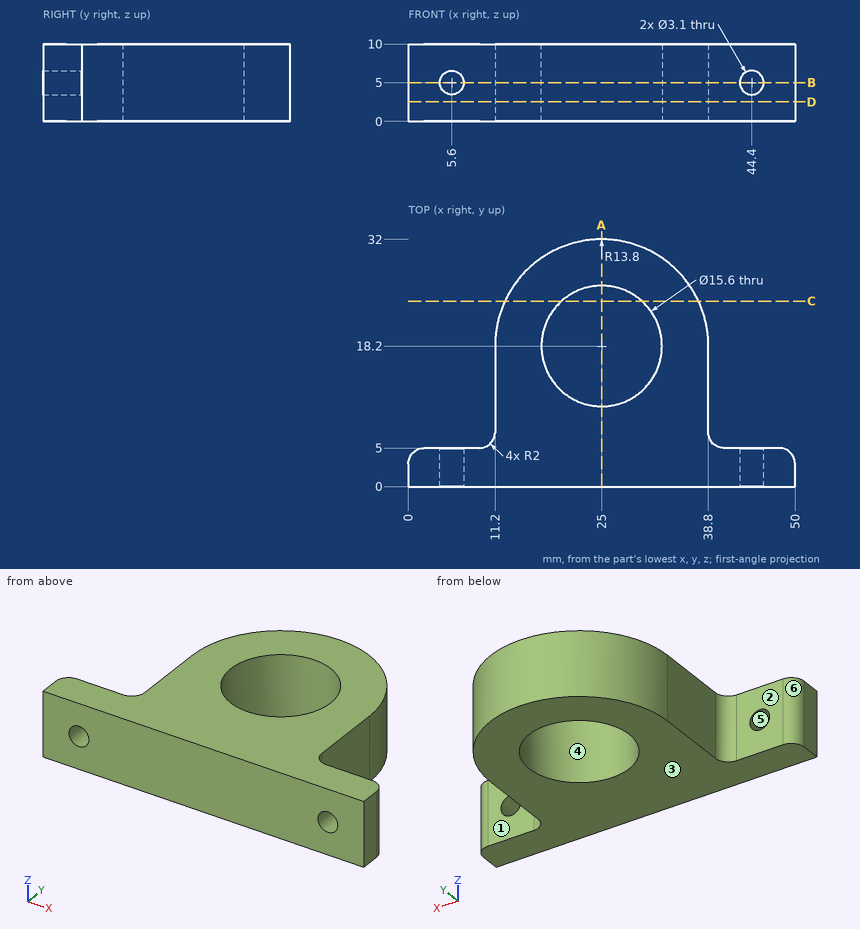
Here's the drawing with two shaded views (mm, measured from the low corner). I have some questions. A direction names the side the tool comes from. Give positions to 0.01 mm unless a question says otherwise; leave off trailing zeros. Order: outer loops, then holes, each group sorted by start corner. A loop starts at its lowest first (then second) coordinate and runs counter-clockwise, first axis right, second up. Notation, with made-up numbers: (50, 58) -> (71, 58) arc R32 ccw to (71, 95) -> close; hole circle Ø7 at (73.5, -30.75). An arc over 180 degrees is marked (long way). One line per item, written item: value. Start each with the question number.
1. Imagine slicing it at A-A, the plane x = 25. List the corners of the cut face in (y, z) for me.
2. Will these pins go through, and if not, where does the flat tip stop? pin 1 Ø1 at (y, z) = (5, 6.5) entering from -X; pin 2 Ø5 at (y, z) = (28, 6) entering from +X; pin 3 Ø3 at (y, z) = (13, 5.5) entering from -X.
3. I need wall thicknesses on probe 1 along X at (y, z) = (1.95, 5); probe 2 along Y at (x, z) = (25, 6.75); probe 3 along X at (y, z) = (18.5, 2.25). Which ranges of each line are inside material? Lowest first, please. Write a range as from..to.
4. For the marked faces 1, 2 and 3, which set-ups out of +Z, -Z, +X, -X, +Y, -Y let a thin tool reach every point of the face, with its end or its side?
5. Imagine slicing it at B-B, the plane z = 5. List the corners of the cut face in (x, y) for me, plus the area to 3 significant figures.
6. Imagine slicing it at D-D, the plane z = 2.5. List the corners of the cut face in (x, y) for me.
7. We'd pull the mould along Y, two halves only. Please class the marked faces 4, 5 and 6: released by +Y, released by -Y, zero draft, split by the parting line, or undercut.
8. Imagine slicing it at C-C, the plane y = 24. List the corners of the cut face in (x, z) for me.
Values follow:
1. outline: (0, 0) -> (10.4, 0) -> (10.4, 10) -> (0, 10) -> close; (26, 0) -> (32, 0) -> (32, 10) -> (26, 10) -> close
2. pin 1: stops at x = 0.68
2. pin 2: stops at x = 36.71
2. pin 3: stops at x = 11.2
3. probe 1: x = 0..4.05, 7.15..42.85, 45.95..50
3. probe 2: y = 0..10.4, 26..32
3. probe 3: x = 11.2..17.21, 32.79..38.8
4. face 1: +Z, -Z, +X, +Y
4. face 2: +Z, -Z, -X, +Y
4. face 3: -Z, +X, -X, +Y, -Y
5. outline: (0, 0) -> (4.05, 0) -> (4.05, 5) -> (2, 5) arc R2 ccw to (0, 3) -> close; (7.15, 0) -> (42.85, 0) -> (42.85, 5) -> (40.8, 5) arc R2 cw to (38.8, 7) -> (38.8, 18.2) arc R13.8 ccw to (11.2, 18.2) -> (11.2, 7) arc R2 cw to (9.2, 5) -> (7.15, 5) -> close; (45.95, 0) -> (50, 0) -> (50, 3) arc R2 ccw to (48, 5) -> (45.95, 5) -> close; hole circle Ø15.6 at (25, 18.2)
5. area: 691 mm2
6. outline: (0, 0) -> (50, 0) -> (50, 3) arc R2 ccw to (48, 5) -> (40.8, 5) arc R2 cw to (38.8, 7) -> (38.8, 18.2) arc R13.8 ccw to (11.2, 18.2) -> (11.2, 7) arc R2 cw to (9.2, 5) -> (2, 5) arc R2 ccw to (0, 3) -> close; hole circle Ø15.6 at (25, 18.2)
7. face 4: undercut
7. face 5: zero draft
7. face 6: released by +Y
8. outline: (12.48, 0) -> (19.78, 0) -> (19.78, 10) -> (12.48, 10) -> close; (30.22, 0) -> (37.52, 0) -> (37.52, 10) -> (30.22, 10) -> close
